For this review, take the finished solid that the model builds, in its own axes (mm). A direction names the side the tool comes from. Give positions to 0.01 mm unless a question says otherwise; leave off trailing zeros. Order: outer loops, then holes, each group sorted by start corner. A loop starts at its lowest first (then second) coordinate and runs counter-clockwise, first axis right, second up.
Item 1: Machinability: for faces 4 (the cylindrical face through (11.695, -36.487, 1.014)), 5 (the flat face through (12, -38, 3)), 6 (the flat face through (11.5, -0.5, 5)), which of the approach directions +Z, -Z, +X, -X, +Y, -Y give a long, thin tool a straight path to every point of the face, cutting with its end or side? Answer none if there is none.
Item 2: Consider section D-D (y = -20). Give the boundary of the cut face in (x, z), plus the area to 4 significant figures.
Item 3: Consider section A-A (z = 10). Give the boundary of the cut face in (x, y), plus the area to 3 significant figures.
Item 4: For P1, Ø2.5, axis at y = -18, z = 14, coming from the +X side; P2, Ø6, axis at y = -33.5, z = 12.5, coming from the -X side; P3, Ø1.5, axis at y = -23.5, z = 3.5, coming from the +X side; P4, Ø4, axis at x = 11.5, y = -20, coming from the +Z side, all flat-tipped, find the tip position at first contact; note any pin that passes through.
Item 5: For probe 1 along X at (y, z) = (-30, 0.85); probe 2 along Z at (x, y) = (14, -4); probe 3 along X at (y, z) = (-13.5, 4), list the stretches that pass through material, from the lowest coordinate up.
Item 6: Consider section B-B (y = -30). Give the boundary of the cut face in (x, z), plus the area to 4 significant figures.
Item 7: The part is to be moulded in two halves that separate along Y. For faces 1 (the flat face through (14.5, -0.5, 2.5)), 2 (the cylindrical face through (12.7, -4.1, 1)), 3 (the flat face through (11.5, -39.5, 5)), say which applies: released by +Y, released by -Y, zero draft, split by the parting line, or undercut.
Item 8: Consider section C-C (x = 3.75). Give the boundary of the cut face in (y, z).
```python
from build123d import *

# Parameters (mm, degrees)
PAD_DEPTH         = 40
SKETCH001_R       = 1.3
POCKET_DEPTH      = 5
CHAMFER_SIZE      = 3
CHAMFER001_SIZE   = 4
SKETCH002_R       = 1.5
POCKET001_DEPTH   = 5.001
POCKET001_FACE6_W = 40
POCKET001_FACE6_H = 7
POCKET001_FACE6_R = 1.5
POCKET008_DEPTH   = 3
SKETCH013_W       = 7
SKETCH013_H       = 2
PAD006_DEPTH      = 3
CHAMFER010_SIZE   = 1
CHAMFER011_SIZE   = 1


with BuildPart() as part:
    # Sketch → Pad (new body)
    with BuildSketch(Plane.XZ):
        Polygon((0, 0), (0, 20), (5, 20), (5, 5), (15, 5), (15, 0), align=None)
    extrude(amount=PAD_DEPTH)

    # Sketch001 (on Face1 of Pad) → Pocket (cut)
    with BuildSketch(Plane(origin=(0, 0, 0), x_dir=(0, 0, -1), z_dir=(-1, 0, 0))):
        with Locations((-10, 30)):
            Circle(SKETCH001_R)
        with Locations((-10, 10)):
            Circle(SKETCH001_R)
    extrude(amount=-POCKET_DEPTH, mode=Mode.SUBTRACT)

    # Chamfer
    chamfer_edges = [part.edges().sort_by_distance(p)[0] for p in [
        (5, -20, 5),
    ]]
    chamfer(chamfer_edges, length=CHAMFER_SIZE)

    # Chamfer001
    chamfer001_edges = [part.edges().sort_by_distance(p)[0] for p in [
        (5, -20, 20),
    ]]
    chamfer(chamfer001_edges, length=CHAMFER001_SIZE)

    # Sketch002 (on Face6 of Chamfer001) → Pocket001 (cut, through all)
    with BuildSketch(Plane(origin=(0, 0, 5), x_dir=(-1, 0, 0), z_dir=(0, 0, 1))):
        with Locations((-11.5, 35)):
            Circle(SKETCH002_R)
        with Locations((-11.5, 30)):
            Circle(SKETCH002_R)
        with Locations((-11.5, 25)):
            Circle(SKETCH002_R)
        with Locations((-11.5, 20)):
            Circle(SKETCH002_R)
        with Locations((-11.5, 15)):
            Circle(SKETCH002_R)
        with Locations((-11.5, 10)):
            Circle(SKETCH002_R)
        with Locations((-11.5, 5)):
            Circle(SKETCH002_R)
    extrude(amount=-POCKET001_DEPTH, mode=Mode.SUBTRACT)

    # Pocket001 Face6 → Pocket008 (cut)
    with BuildSketch(Plane(origin=(11.5, -20, 5), x_dir=(0, 1, 0), z_dir=(0, 0, 1))):
        Rectangle(POCKET001_FACE6_W, POCKET001_FACE6_H)
        with Locations((-15, 0)):
            Circle(POCKET001_FACE6_R, mode=Mode.SUBTRACT)
        with Locations((-10, 0)):
            Circle(POCKET001_FACE6_R, mode=Mode.SUBTRACT)
        with Locations((-5, 0)):
            Circle(POCKET001_FACE6_R, mode=Mode.SUBTRACT)
        Circle(POCKET001_FACE6_R, mode=Mode.SUBTRACT)
        with Locations((5, 0)):
            Circle(POCKET001_FACE6_R, mode=Mode.SUBTRACT)
        with Locations((10, 0)):
            Circle(POCKET001_FACE6_R, mode=Mode.SUBTRACT)
        with Locations((15, 0)):
            Circle(POCKET001_FACE6_R, mode=Mode.SUBTRACT)
    extrude(amount=-POCKET008_DEPTH, mode=Mode.SUBTRACT)

    # Sketch013 (on Face7 of Pocket008) → Pad006 (join)
    with BuildSketch(Plane(origin=(0, 0, 2), x_dir=(-1, 0, 0), z_dir=(0, 0, 1))):
        with Locations((-11.5, 39)):
            Rectangle(SKETCH013_W, SKETCH013_H)
        with Locations((-11.5, 1)):
            Rectangle(SKETCH013_W, SKETCH013_H)
    extrude(amount=PAD006_DEPTH)

    # Chamfer010
    chamfer010_edges = [part.edges().sort_by_distance(p)[0] for p in [
        (15, -40, 2.5),
        (15, 0, 2.5),
    ]]
    chamfer(chamfer010_edges, length=CHAMFER010_SIZE)

    # Chamfer011
    chamfer011_edges = [part.edges().sort_by_distance(p)[0] for p in [
        (11.5, -2, 5),
        (11.5, -38, 5),
    ]]
    chamfer(chamfer011_edges, length=CHAMFER011_SIZE)


solid = part.part
```
Resolved:
1. face 4: +Z, -Z
1. face 5: +Z, +X
1. face 6: +Z, +X, +Y, -Y
2. outline: (0, 0) - (10, 0) - (10, 2) - (8, 2) - (8, 5) - (5, 8) - (5, 16) - (1, 20) - (0, 20) - close; (13, 0) - (15, 0) - (15, 2) - (13, 2) - close
2. area: 119.5 mm2
3. outline: (0, -40) - (5, -40) - (5, -31.3) - (0, -31.3) - close; (0, -28.7) - (5, -28.7) - (5, -11.3) - (0, -11.3) - close; (0, -8.7) - (5, -8.7) - (5, 0) - (0, 0) - close
3. area: 174 mm2
4. P1: stops at x = 5
4. P2: stops at x = 0
4. P3: stops at x = 8
4. P4: stops at z = 2
5. probe 1: x = 0 to 10, 13 to 15
5. probe 2: z = 0 to 2
5. probe 3: x = 0 to 8
6. outline: (0, 0) - (10, 0) - (10, 2) - (8, 2) - (8, 5) - (5, 8) - (5, 8.7) - (0, 8.7) - close; (0, 11.3) - (5, 11.3) - (5, 16) - (1, 20) - (0, 20) - close; (13, 0) - (15, 0) - (15, 2) - (13, 2) - close
6. area: 106.5 mm2
7. face 1: released by +Y
7. face 2: undercut
7. face 3: zero draft
8. outline: (-40, 0) - (0, 0) - (0, 17.25) - (-40, 17.25) - close; hole circle Ø2.6 at (-30, 10); hole circle Ø2.6 at (-10, 10)
